from build123d import *

# Parameters (mm, degrees)
F0_R     = 15
F1_DEPTH = 5
F2_R     = 5
F3_DEPTH = 50
F5_D     = 5.5


with BuildPart() as f1:
    # F0 (on Front) → F1 (new body)
    with BuildSketch(Plane.XZ):
        Circle(F0_R)
    extrude(amount=F1_DEPTH)

    # F2 (on face) → F3 (join)
    with BuildSketch(Plane.XZ.offset(5)):
        Circle(F2_R)
    extrude(amount=F3_DEPTH)

    # F5 (through all)
    with Locations(Plane.XZ.offset(55)):
        with Locations((0, 0)):
            Hole(F5_D / 2)


solid = f1.part
Work out the finished part from the listing and answer in its coordinate system (mm). A direction names the side the tool comes from. Round coordinates to 2 decimals unless told otherwise and drop trailing zeros. Write each loop counter-clockwise with the first axis right and the second up, starting at its lowest first coordinate (ties: lowest second). Pieces come first, ordered by that corner, then holes.
1) A cutting plane is placed at D-D (x = 4.25). Give the vertices of the cut face in (y, z).
2) A tool of negligible diameter and unlimited length cuts with its end or side. For faces 1 (the flat face through (2.2, -55, -2.2)), 2 (the cylindrical face through (-1.08, -29.65, -4.88)), from which of +Z, -Z, +X, -X, +Y, -Y can it reach the whole face along a straight path? Write none if from no direction.
3) A cutting plane is placed at A-A (x = 0). Give the vertices of the cut face in (y, z), plus the area to 4 significant figures.
4) Given pin 1 Ø6 at (y, z) = (-28.5, 6) entering from +X; pin 2 Ø5 at (x, z) = (-1.5, -7.5) entering from +Y; pin 3 Ø2 at (y, z) = (-11, 1.5) entering from +X; pin 4 Ø1.5 at (x, z) = (-9.5, -7) entering from -Y, each flat-ended and moving along its own axis, determine where each tip first touches the part or whether it passes through.
5) A cutting plane is placed at C-C (y = -39). Give the vertices of the cut face in (x, z).
6) Straight lines are drawn through the part: line 1 (Z direction, x = 0, y = -34.5); line 2 (Y direction, x = -7, z = -9.75); line 3 (X direction, y = -11, z = -1.5). For each, find the intervals that lie inside material, in ascending order.
7) A cutting plane is placed at B-B (z = 0). Give the vertices of the cut face in (x, y), plus the area to 4 significant figures.
8) The mould has two halves that part along X. Classify faces 3 (the cylindrical face through (0.596, -27.115, -2.685)), 4 (the cylindrical face through (-14.985, -2.465, 0.66)), 5 (the flat face through (3, 0, 0)): pulls with the +X half, pulls with the -X half, needs draft (parallel to the pull), parting line crosses it, or undercut.
Completed:
1. outline: (-55, -2.63) - (-5, -2.63) - (-5, -14.39) - (0, -14.39) - (0, 14.39) - (-5, 14.39) - (-5, 2.63) - (-55, 2.63) - close
2. face 1: +Z, -Z, +X, -X, -Y
2. face 2: -Y
3. outline: (-55, -5) - (-5, -5) - (-5, -15) - (0, -15) - (0, -2.75) - (-55, -2.75) - close; (-55, 2.75) - (0, 2.75) - (0, 15) - (-5, 15) - (-5, 5) - (-55, 5) - close
3. area: 347.5 mm2
4. pin 1: stops at x = 4
4. pin 2: stops at y = 0
4. pin 3: stops at x = 4.97
4. pin 4: stops at y = -5
5. outline: circle Ø10 at (0, 0); hole circle Ø5.5 at (0, 0)
6. line 1: z = -5 to -2.75, 2.75 to 5
6. line 2: y = -5 to 0
6. line 3: x = -4.77 to -2.3, 2.3 to 4.77
7. outline: (-15, -5) - (-5, -5) - (-5, -55) - (-2.75, -55) - (-2.75, 0) - (-15, 0) - close; (2.75, -55) - (5, -55) - (5, -5) - (15, -5) - (15, 0) - (2.75, 0) - close
7. area: 347.5 mm2
8. face 3: undercut
8. face 4: parting line crosses it
8. face 5: needs draft
